```python
from build123d import *

# Parameters (mm, degrees)
F0_W      = 19.67
F0_H      = 14.05
F0_R      = 4.25
F1_DEPTH  = 6.5
F2_DEPTH  = 15.5
F3_R      = 5
F4_DEPTH  = 2.78
F5_W      = 7.1
F5_H      = 10.22
F6_DEPTH  = 2.9
F7_W      = 5.5
F7_H      = 2
F8_DEPTH  = 5.5
F10_DEPTH = 31


with BuildPart() as f1:
    # F0 (on Front) → F1 (new body)
    with BuildSketch(Plane.XZ):
        with Locations((9.835, -7.025)):
            Rectangle(F0_W, F0_H)
        with Locations((9.835, -7.025)):
            Circle(F0_R, mode=Mode.SUBTRACT)
        with Locations((9.835, -7.025)):
            Circle(F0_R)
    extrude(amount=F1_DEPTH)

    # F0 (on Front) → F2 (join)
    with BuildSketch(Plane.XZ):
        with Locations((9.835, -7.025)):
            Circle(F0_R)
    extrude(amount=F2_DEPTH)

    # F3 (on face) → F4 (join)
    with BuildSketch(Plane.XZ.offset(15.5)):
        with Locations((9.835, -7.025)):
            Circle(F3_R)
    extrude(amount=-F4_DEPTH)

    # F5 (on face) → F6 (join)
    with BuildSketch(Plane(origin=(0, 0, 0), x_dir=(-1, 0, 0), z_dir=(0, 1, 0))):
        with Locations((-16.12, -5.11)):
            Rectangle(F5_W, F5_H)
    extrude(amount=F6_DEPTH)

    # F7 (on face) → F8 (join)
    with BuildSketch(Plane.XY):
        with Locations((8.45, -1)):
            Rectangle(F7_W, F7_H)
    extrude(amount=F8_DEPTH)

    # F9 (on face) → F10 (join)
    with BuildSketch(Plane.XY.offset(5.5)):
        with BuildLine():
            ThreePointArc((8.45, 0), (7.813604, -1.536396), (9.35, -0.9))
            ThreePointArc((9.35, -0.9), (9.086396, -0.263604), (8.45, 0))
        make_face()
    extrude(amount=F10_DEPTH)


solid = f1.part
```
Work out the finished part from the listing and answer in its coordinate system (mm). A direction names the side the tool comes from. Give positions to 0.01 mm unless a question says otherwise; leave off trailing zeros. Loops run counter-clockwise (first coordinate to the right, second up) from the corner with the lowest first, then second, coordinate; pieces in that order, holes last. Notation, with made-up numbers: (25, 56) -> (61, 56) arc R16 cw to (61, 73) -> close; hole circle Ø11 at (10, -29). An arc over 180 degrees is marked (long way). Write item = value, one per line. Start each with the question number.
(1) Find the intervals of material crossed by probe 1 along Y at (x, z) = (5.5, -6); probe 2 along Z at (x, y) = (18.75, -3); probe 3 along Z at (x, y) = (12.75, 1.25), in increasing order. Write a range as from..to.
(2) Which of the six approach directions +Z, -Z, +X, -X, +Y, -Y give full straight-line access (tool end or side, diameter ignored) to faces 1 (the flat face through (12.57, 1, -5)), 2 (the flat face through (16, 1, -10.22)), 3 (the flat face through (8, -2, 3)), 4 (the flat face through (5.7, -1, 3)), 5 (the cylindrical face through (8.751, -14.129, -11.906))?
(3) Find section D-D on x = 2.5. Give the vertices of the cut face in (y, z).
(4) Find section C-C on z = 13.5. Give the vertices of the cut face in (x, y).
(5) Find section B-B on y = 1. Give the vertices of the cut face in (x, z), and give its area (3 significant figures).
(6) The mould has two halves that part along Y. Classify faces 6 (the cylindrical face through (5.59, -9.57, -6.84)), 7 (the flat face through (10, -15.5, -7)), 8 (the flat face through (12, -12.72, -11)), 9 (the flat face through (11.2, -1, 3)): +Y half, -Y half, draft (parallel to the pull), parting line (faces both ways), or undercut.
(7) Find section A-A on x = 16.75. Give the vertices of the cut face in (y, z).
(8) Given pin 1 Ø3 at (y, z) = (2, -6.5) entering from -X; pin 2 Ø4 at (y, z) = (-1.5, 17) entering from -X; pin 3 Ø8 at (x, z) = (5.5, 26.5) entering from +Y; pin 4 Ø1.5 at (x, z) = (11.5, 18.5) entering from -Y, each flat-ended and moving along its own axis, determine where each tip first touches the part or whether it passes through.
From the geometry:
q1.probe_1 = -15.5..-12.72, -6.5..0
q1.probe_2 = -14.05..0
q1.probe_3 = -10.22..0
q2.face_1 = +Z, -Z, -X, +Y
q2.face_2 = -Z, +X, -X, +Y
q2.face_3 = +Z, +X, -X, -Y
q2.face_4 = +Z, -X, +Y, -Y
q2.face_5 = -Y
q3.outline = (-6.5, -14.05) -> (0, -14.05) -> (0, 0) -> (-6.5, 0) -> close
q4.outline = circle Ø1.8 at (8.45, -0.9)
q5.outline = (12.57, -10.22) -> (19.67, -10.22) -> (19.67, 0) -> (12.57, 0) -> close
q5.area = 72.6 mm^2
q6.face_6 = undercut
q6.face_7 = -Y half
q6.face_8 = undercut
q6.face_9 = draft
q7.outline = (-6.5, -14.05) -> (0, -14.05) -> (0, -10.22) -> (2.9, -10.22) -> (2.9, 0) -> (-6.5, 0) -> close
q8.pin_1 = 12.57
q8.pin_2 = 7.55
q8.pin_3 = 0
q8.pin_4 = through
